The model under review builds one solid part; all positions refer to its coordinate system, in mm. A direction names the side the tool comes from. Coordinates: 2 decimals unless noted, no trailing zeros. Loops run counter-clockwise (first coordinate to the right, second up) from the corner with the lowest first, then second, coordinate; pieces in that order, holes last. Notation, with made-up numbers: M 54,8 L 82,8 A28 cw 82,29 Z; hole C 78,56.5 d5. An arc over 180 degrees is marked long. Use CSV: the item, a comma, the result in double quotes. Start each with the question number.
1. Add section A-A, the plane y = 0. Write out the cut boundary in (x, z).
2. Tool access review of faces 4 (the cylindrical face through (10.418, -3.281, 3.757)), 5 (the flat face through (14, 0, 9.652)): name each direction out of +Z, -Z, +X, -X, +Y, -Y from which nothing blocks a thin tool from reaching the whole face with its end or side.
3. For L1, parallel to Y at x = 0, z = 8.85; L2, parallel to Y at x = -3, z = 7.5; L3, parallel to Z at x = -16, y = -22.5, list the stretches that pass through material, from the lowest coordinate up.
4. Add section C-C, the plane z = 5.25. Write out the cut boundary in (x, y).
5. Add section D-D, the plane x = -12.5. Write out the cut boundary in (y, z).
6. Clearance check with flat-ended pins moving along their axes: P1, Ø1, axis at x = -5.5, y = 7.5, coming from the -Z side; P2, Ø1.5, axis at y = 4, z = 8.5, coming from the +X side; P3, Ø1, axis at x = 17, z = 2, coming from the -Y side. State where each tip first meets the part, or that it passes through.
7. Draft analysis for pull direction Y (two halves, no side actions). For faces 1 (the cylindrical face through (-10.418, 3.281, 9.008)), 2 (the flat face through (12, 0, 0)), 3 (the cylindrical face through (-6.883, -30.995, 8.364)), state which applies: +Y half, -Y half, draft (parallel to the pull), parting line (faces both ways), or undercut.
from build123d import *

# Parameters (mm, degrees)
F0_R           = 27.178
F1_DEPTH       = 7.112
F2_R           = 31.75
F3_DEPTH       = 2.54
F5_D           = 19.304
F5_DEPTH       = 7.62
F5_CBORE_D     = 21.844
F5_CBORE_DEPTH = 7.62
F5_TIP         = 5.7995066949
F7_D           = 21.844
F7_DEPTH       = 1.27
F7_TIP         = 6.562599681


with BuildPart() as f1:
    # F0 (on Top) → F1 (new body)
    with BuildSketch(Plane.XY):
        Circle(F0_R)
    extrude(amount=F1_DEPTH)

    # F2 (on face) → F3 (join)
    with BuildSketch(Plane.XY.offset(7.112)):
        Circle(F2_R)
    extrude(amount=F3_DEPTH)

    # F5
    with Locations(Plane(origin=(0, 0, 0), x_dir=(1, 0, 0), z_dir=(0, 0, -1))):
        with Locations((0, 0)):
            CounterBoreHole(F5_D / 2, F5_CBORE_D / 2, F5_CBORE_DEPTH, depth=F5_DEPTH)
            with Locations((0, 0, -(F5_DEPTH + F5_TIP / 2))):  # 118° drill point
                Cone(0, F5_D / 2, F5_TIP, mode=Mode.SUBTRACT)

    # F7
    with Locations(Plane.XY.offset(9.652)):
        with Locations((0, 0)):
            Hole(F7_D / 2, depth=F7_DEPTH)
            with Locations((0, 0, -(F7_DEPTH + F7_TIP / 2))):  # 118° drill point
                Cone(0, F7_D / 2, F7_TIP, mode=Mode.SUBTRACT)


solid = f1.part
Computed:
1,outline,"M -31.75,7.11 L -27.18,7.11 L -27.18,0 L -10.92,0 L -10.92,7.62 L -9.65,7.62 L -10.92,8.38 L -10.92,9.65 L -31.75,9.65 Z; M 9.65,7.62 L 10.92,7.62 L 10.92,0 L 27.18,0 L 27.18,7.11 L 31.75,7.11 L 31.75,9.65 L 10.92,9.65 L 10.92,8.38 Z"
2,face 4,"-Z"
2,face 5,"+Z, +X, -X, +Y, -Y"
3,L1,"y = -31.75 to -10.92, 10.92 to 31.75"
3,L2,"y = -31.61 to -10.5, 10.5 to 31.61"
3,L3,"z = 7.11 to 9.65"
4,outline,"C 0,0 d54.36; hole C 0,0 d21.84"
5,outline,"M -29.19,7.11 L -24.13,7.11 L -24.13,0 L 24.13,0 L 24.13,7.11 L 29.19,7.11 L 29.19,9.65 L -29.19,9.65 Z"
6,P1,"stops at z = 7.62"
6,P2,"stops at x = 31.58"
6,P3,"stops at y = -21.6"
7,face 1,"undercut"
7,face 2,"draft"
7,face 3,"parting line"
